Build history of the part. All positions in model axes, mm. Give positions to 0.01 mm unless a question says otherwise; leave off trailing zeros. Order: outer loops, then holes, each group sorted by start corner. A loop starts at its lowest first (then second) coordinate and runs counter-clockwise, first axis right, second up. Notation, with made-up numbers: (87.25, 7) - (119.25, 7) arc R21 cw to (119.25, 46) - close; hole circle Ø10 at (82.5, 77). An arc over 180 degrees is marked (long way). Use a Markdown table: item, result.
from build123d import *

# Parameters (mm, degrees)
BOSS_EXTRUDE1_DEPTH      = 1.5875
BOSS_EXTRUDE1_DEPTH_BACK = 1.5875
CUT_EXTRUDE2_DEPTH       = 284.597068155
BOSS_EXTRUDE2_DEPTH      = 3.175
FILLET1_R                = 6.35
FILLET2_R                = 6.35


with BuildPart() as part:
    # CS path → Boss-Extrude1 (new, two sides: drawn at the far end of the back side and taken through both)
    with BuildSketch(Plane(origin=(0, 0, 0), x_dir=(1, 0, 0), z_dir=(0, 1, 0)).offset(-BOSS_EXTRUDE1_DEPTH_BACK)):
        Polygon((-228.6, 0), (228.6, 0), (0, -163.068), (-127, -163.068), align=None)
    extrude(amount=BOSS_EXTRUDE1_DEPTH + BOSS_EXTRUDE1_DEPTH_BACK)

    # Sweep1: sweep along a curve in space
    with BuildLine() as sweep1_path:
        Line((-228.6, 1.5875, 0), (-127, 1.5875, 163.068))
    # Sketch10 → Sweep1 (sweep)
    with BuildSketch(Plane.XY.offset(163.068)):
        Polygon((-127, 1.5875), (-130.404404736, 0), (-127, -1.5875), align=None)
    sweep(path=sweep1_path.line)

    # Sweep2: sweep along a curve in space
    with BuildLine() as sweep2_path:
        Line((0, 1.5875, 163.068), (228.6, 1.5875, 0))
    # Sketch11 → Sweep2 (sweep)
    with BuildSketch(Plane.XY.offset(163.068)):
        Polygon((0, 1.5875), (3.404404736, 0), (0, -1.5875), align=None)
    sweep(path=sweep2_path.line)

    # Sketch2 → Cut-Extrude2 (cut, through all)
    with BuildSketch(Plane(origin=(0, 1.5875, 0), x_dir=(1, 0, 0), z_dir=(0, 1, 0))):
        Polygon((-205.723873178, -12.7), (188.927034488, -12.7), (-4.065488877, -150.368), (-119.94941835, -150.368), align=None)
    extrude(amount=-CUT_EXTRUDE2_DEPTH, mode=Mode.SUBTRACT)

    # Sketch3 → Boss-Extrude2 (add)
    with BuildSketch(Plane(origin=(0, 1.5875, 0), x_dir=(1, 0, 0), z_dir=(0, 1, 0))):
        Polygon((-8.215599111, -12.7), (-121.714648415, -147.534805746), (-119.94941835, -150.368), (-115.799308116, -150.368), (-7.240488877, -21.402097696), (-7.240488877, -150.368), (-4.065488877, -150.368), (-0.890488877, -148.103166667), (-0.890488877, -18.864845516), (89.697119406, -83.484006092), (95.164426205, -79.583993908), (1.401817922, -12.7), align=None)
    extrude(amount=-BOSS_EXTRUDE2_DEPTH)

    # Fillet1
    fillet1_edges = [part.edges().sort_by_distance(p)[0] for p in [
        (-7.240488877, 0, 150.368),
        (-7.240488877, 0, 21.402097696),
        (-115.799308116, 0, 150.368),
        (-121.714648415, 0, 147.534805746),
        (-8.215599111, 0, 12.7),
        (1.401817922, 0, 12.7),
        (95.164426205, 0, 79.583993908),
        (89.697119406, 0, 83.484006092),
        (-0.890488877, 0, 18.864845516),
        (-0.890488877, 0, 148.103166667),
    ]]
    fillet(fillet1_edges, radius=FILLET1_R)

    # Fillet2
    fillet2_edges = [part.edges().sort_by_distance(p)[0] for p in [
        (-205.723873178, 0, 12.7),
        (188.927034488, 0, 12.7),
    ]]
    fillet(fillet2_edges, radius=FILLET2_R)


solid = part.part
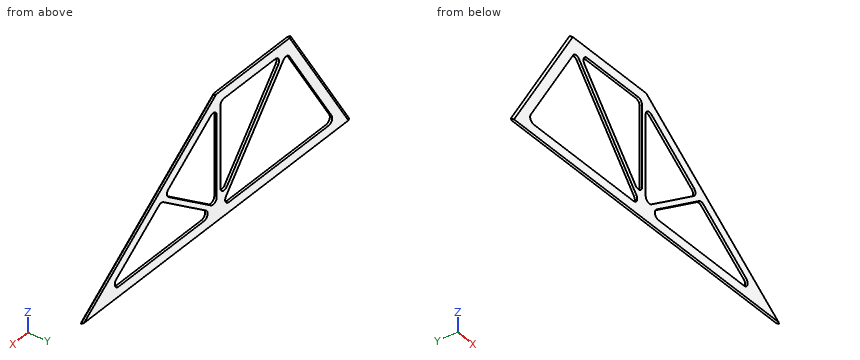
1) Slice it at C-C (z = 44). Write the cut outline in (x, y), and give its area (3 significant figures).
Computed:
| item | result |
|---|---|
| outline | (-204.59, 0) - (-201.19, -1.59) - (-186.22, -1.59) - (-186.22, 1.59) - (-201.19, 1.59) - close; (-34.56, -1.59) - (-26.26, -1.59) - (-26.26, 1.59) - (-34.56, 1.59) - close; (-7.24, -1.59) - (-0.89, -1.59) - (-0.89, 1.59) - (-7.24, 1.59) - close; (34.35, -1.59) - (45.28, -1.59) - (45.28, 1.59) - (34.35, 1.59) - close; (145.05, -1.59) - (166.92, -1.59) - (170.32, 0) - (166.92, 1.59) - (145.05, 1.59) - close |
| area | 209 mm² |
2) Slice it at B-B (y = 0.6). State how many separate pieces and enclosed holes the cut face has, and give its area (3 significant figures).
Computed:
| item | result |
|---|---|
| separate pieces | 1 |
| enclosed holes | 4 |
| area | 16,300 mm² |
3) Slice it at D-D (x = -155). Write the cut outline in (y, z).
Computed:
| item | result |
|---|---|
| outline | (-1.59, 0) - (1.59, 0) - (1.59, 12.7) - (-1.59, 12.7) - close; (-1.59, 94.11) - (1.59, 94.11) - (1.59, 118.13) - (0, 123.59) - (-1.59, 118.13) - close |
4) Pin check, flat tips, straight feed: P1, Ø1.5, axis at x = 99, y = -0.5, coming from the +Z side; P2, Ø1.6, axis at x = 62, y = -0.5, coming from the +Z side; P3, Ø1, axis at y = -0.5, z = 72.5, coming from the -X side. Stop position of each tip, or through.
Computed:
| item | result |
|---|---|
| P1 | stops at z = 95.28 |
| P2 | stops at z = 121.72 |
| P3 | stops at x = -186.88 |
5) Wall check: line 1 (X direction, y = -0.65, z = 102.5); line 2 (X direction, y = -0.85, z = 120); line 3 (Z direction, x = 24, y = 0.6). Give the ranges that are in metal, low to high. Write a range as from..to.
Computed:
| item | result |
|---|---|
| line 1 | x = -166.75..-149.77, -83.81..-75.51, -7.24..-0.89, 63.04..86.92 |
| line 2 | x = -155.42..-138.87, -98.54..-90.24, -7.24..-0.89, 38.51..61.96 |
| line 3 | z = 0..12.7, 28.82..36.62, 130.35..147.46 |
6) Slice it at A-A (x = -88.5). Write the cut outline in (y, z).
Computed:
| item | result |
|---|---|
| outline | (-1.59, 0) - (1.59, 0) - (1.59, 12.7) - (-1.59, 12.7) - close; (-1.59, 108.08) - (1.59, 108.08) - (1.59, 117.94) - (-1.59, 117.94) - close; (-1.59, 150.37) - (1.59, 150.37) - (1.59, 163.07) - (-1.59, 163.07) - close |
